from build123d import *

# Parameters (mm, degrees)
SKETCH1_R           = 2.5
BOSS_EXTRUDE1_DEPTH = 3.1


with BuildPart() as part:
    # Sketch1 → Boss-Extrude1 (new body)
    with BuildSketch(Plane.XY):
        Polygon((20, -25.484827557), (24.75, -22.742413779), (24.75, -17.257586221), (20, -14.515172443), (15.25, -17.257586221), (15.25, -22.742413779), align=None)
        with Locations(Location((20, -20, 0), (0, 0, 180))):
            Circle(SKETCH1_R, mode=Mode.SUBTRACT)
    extrude(amount=BOSS_EXTRUDE1_DEPTH)


solid = part.part
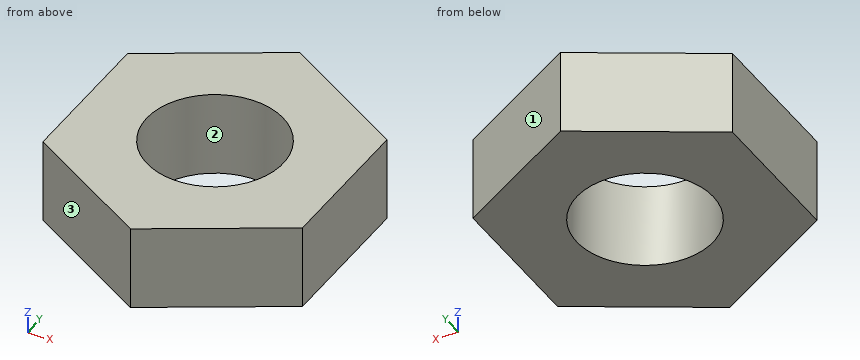
Input: part model. Units: mm. Frame: model coordinates. Face numbers are marked on the shaded views. Coordinates: 2 decimals unless noted, no trailing zeros. Loops run counter-clockwise (first coordinate to the right, second up) from the corner with the lowest first, then second, coordinate; pieces in that order, holes last. Notation, with made-up numbers: (74, 10.5) -> (133, 10.5) arc R10 cw to (133, 21.5) -> close; hole circle Ø6 at (-3, -32.5). An arc over 180 degrees is marked (long way). Write item = value, one per line. Start each with the question number.
Item 1: Material intervals for line 1 (X direction, y = -20, z = 2.15); line 2 (X direction, y = -21, z = 0.6); line 3 (Y direction, x = 21.75, z = 1.45), sorted ascending.
Item 2: First-contact query: P1, Ø4, axis at x = 20, y = -20, coming from the +Z side; P2, Ø5, axis at x = 16.5, y = -19.5, coming from the -Z side. Flat tips, straight axial feed; report the tip coordinate or a pass-through.
Item 3: Cut plane D-D, the plane x = 24.25. Return loops of the section in (y, z).
Item 4: Cut plane C-C, the plane z = 2.4. Return loops of the section in (x, y), plus the area to 3 significant figures.
Item 5: Mould query, pull axis X, two halves, no side actions, for the marked faces 1, 2 and 3. Classes: pulls with the +X half, pulls with the -X half, needs draft (parallel to the pull), parting line crosses it, or undercut.
Item 6: Cut plane B-B, the plane x = 21.5. Return loops of the section in (y, z).
Item 7: Cut plane A-A, the plane y = -20. Return loops of the section in (x, z), plus the area to 4 significant figures.
Ans:
q1.line_1 = 15.25 to 17.5, 22.5 to 24.75
q1.line_2 = 15.25 to 17.71, 22.29 to 24.75
q1.line_3 = -24.47 to -21.79, -18.21 to -15.53
q2.P1 = through
q2.P2 = 0
q3.outline = (-23.03, 0) -> (-16.97, 0) -> (-16.97, 3.1) -> (-23.03, 3.1) -> close
q4.outline = (15.25, -22.74) -> (20, -25.48) -> (24.75, -22.74) -> (24.75, -17.26) -> (20, -14.52) -> (15.25, -17.26) -> close; hole circle Ø5 at (20, -20)
q4.area = 58.5 mm²
q5.face_1 = pulls with the +X half
q5.face_2 = undercut
q5.face_3 = pulls with the -X half
q6.outline = (-24.62, 0) -> (-22, 0) -> (-22, 3.1) -> (-24.62, 3.1) -> close; (-18, 0) -> (-15.38, 0) -> (-15.38, 3.1) -> (-18, 3.1) -> close
q7.outline = (15.25, 0) -> (17.5, 0) -> (17.5, 3.1) -> (15.25, 3.1) -> close; (22.5, 0) -> (24.75, 0) -> (24.75, 3.1) -> (22.5, 3.1) -> close
q7.area = 13.95 mm²
